CAD build for the part. Positions are in the model's coordinates, mm. Round coordinates to 2 decimals unless told otherwise and drop trailing zeros. Loops run counter-clockwise (first coordinate to the right, second up) from the corner with the lowest first, then second, coordinate; pieces in that order, holes last. Notation, with made-up numbers: M 50,-13 L 94,-13 A24 cw 94,4 Z; hole C -14,-8.5 d2. An arc over 180 degrees is marked long. Put each result on its own line as item: value. Start each with the question number.
from build123d import *

# Parameters (mm, degrees)
SKETCH1_W           = 8.5
SKETCH1_H           = 8
BOSS_EXTRUDE1_DEPTH = 4.2
CUT_EXTRUDE1_DEPTH  = 14.2
CHAMFER1_SIZE       = 1.090756547
CHAMFER1_SIZE_2     = 1
FILLET1_R           = 1
FILLET2_R           = 0.2
FILLET3_R           = 0.02
SKETCH3_R           = 0.5
CUT_EXTRUDE2_DEPTH  = 14.2
CHAMFER2_SIZE       = 0.1


with BuildPart() as part:
    # Sketch1 → Boss-Extrude1 (new body)
    with BuildSketch(Plane(origin=(0, 0, 0), x_dir=(1, 0, 0), z_dir=(0, 1, 0))):
        Rectangle(SKETCH1_W, SKETCH1_H)
    extrude(amount=BOSS_EXTRUDE1_DEPTH)

    # Sketch2 → Cut-Extrude1 (cut)
    with BuildSketch(Plane(origin=(4.25, 0, 0), x_dir=(0, 0, -1), z_dir=(1, 0, 0))):
        with BuildLine():
            Line((-4, 3.9), (-5.253535024, 5.241651662))
            Line((-5.253535024, 5.241651662), (3.889156526, 7.141243929))
            Line((3.889156526, 7.141243929), (5.679183493, 5.077233243))
            Line((5.679183493, 5.077233243), (4, 3.9))
            ThreePointArc((4, 3.9), (0, 4.060256822), (-4, 3.9))
        make_face()
        with BuildLine():
            Line((4.717394395, 0), (0, -2.904825783))
            Line((0, -2.904825783), (-4.70037365, 0))
            ThreePointArc((-4.70037365, 0), (0.008510373, 0.222229748), (4.717394395, 0))
        make_face()
    extrude(amount=-CUT_EXTRUDE1_DEPTH, mode=Mode.SUBTRACT)

    # Chamfer1
    # the kernel refuses this chamfer: 1.090756547, 1 mm, written as the material it takes off along each edge
    with BuildSketch(Plane(origin=(7.060832105, 3.9, -4), x_dir=(0, -1, 0), z_dir=(-1, 0, 0))) as chamfer1_piece_1:
        with BuildLine():
            Line((CHAMFER1_SIZE, 0), (-0.069441157, 0.98780495))
            ThreePointArc((-0.069441157, 0.98780495), (-0.038234412, 0.508961249), (0, 0))
            Line((0, 0), (CHAMFER1_SIZE, 0))
        make_face()
    extrude(amount=14.12166421, mode=Mode.SUBTRACT)
    with BuildSketch(Plane(origin=(7.026184696, 3.9, 4), x_dir=(0, 0.06925797782051132, -0.9975987833333668), z_dir=(-1, 0, 0))) as chamfer1_piece_2:
        with BuildLine():
            Line((1.077190612, 0), (-CHAMFER1_SIZE_2 * 0.0692579778205, CHAMFER1_SIZE_2 * 0.997598783333))
            Line((-CHAMFER1_SIZE_2 * 0.0692579778205, CHAMFER1_SIZE_2 * 0.997598783333), (0, 0))
            ThreePointArc((0, 0), (0.555048482, -0.002898226), (1.077190612, 0))
        make_face()
    extrude(amount=14.052369392, mode=Mode.SUBTRACT)

    # Fillet1
    fillet1_edges = [part.edges().sort_by_distance(p)[0] for p in [
        (0, 0.062655213, -4),
        (0, 0.061289175, 4),
    ]]
    fillet(fillet1_edges, radius=FILLET1_R)

    # Fillet2
    fillet2_edges = [part.edges().sort_by_distance(p)[0] for p in [
        (0, 2.809243453, -4),
        (0, 3.974604043, 2.925395957),
        (0, 3.969441157, -3.01219505),
        (0, 2.9, 4),
    ]]
    fillet(fillet2_edges, radius=FILLET2_R)

    # Fillet3
    fillet3_edges = [part.edges().sort_by_distance(p)[0] for p in [
        (4.25, 0.222229049, -0.000152397),
        (4.25, 0.406869221, -3.686055151),
        (4.25, 0.405751593, 3.685933525),
        (-4.25, 0.222229049, -0.000152397),
        (-4.25, 0.406869221, -3.686055151),
        (-4.25, 0.405751593, 3.685933525),
        (4.25, 1.93502694, -4),
        (-4.25, 1.93502694, -4),
        (4.25, 1.975286544, 4),
        (4.25, 3.384901314, -3.509878633),
        (4.25, 4.060241686, -0.03890618),
        (4.25, 3.439667659, 3.460332341),
        (4.25, 2.893693974, 3.984775907),
        (4.25, 3.961854563, 2.919594368),
        (4.25, 3.953888859, -3.004346497),
        (4.25, 2.804713491, -3.987691713),
        (-4.25, 3.384901314, -3.509878633),
        (-4.25, 1.975286544, 4),
        (-4.25, 3.439667659, 3.460332341),
        (-4.25, 4.060241686, -0.03890618),
        (-4.25, 2.893693974, 3.984775907),
        (-4.25, 3.961854563, 2.919594368),
        (-4.25, 3.953888859, -3.004346497),
        (-4.25, 2.804713491, -3.987691713),
    ]]
    fillet(fillet3_edges, radius=FILLET3_R)

    # Sketch3 → Cut-Extrude2 (cut)
    with BuildSketch(Plane.ZY.offset(4.25)):
        with Locations((-1.55, 1.4)):
            Circle(SKETCH3_R)
        with Locations((1.55, 1.4)):
            Circle(SKETCH3_R)
    extrude(amount=-CUT_EXTRUDE2_DEPTH, mode=Mode.SUBTRACT)

    # Chamfer2
    chamfer2_edges = [part.edges().sort_by_distance(p)[0] for p in [
        (4.25, 1.4, -2.05),
        (-4.25, 1.4, -2.05),
        (4.25, 1.4, 1.05),
        (-4.25, 1.4, 1.05),
    ]]
    chamfer(chamfer2_edges, length=CHAMFER2_SIZE)


solid = part.part
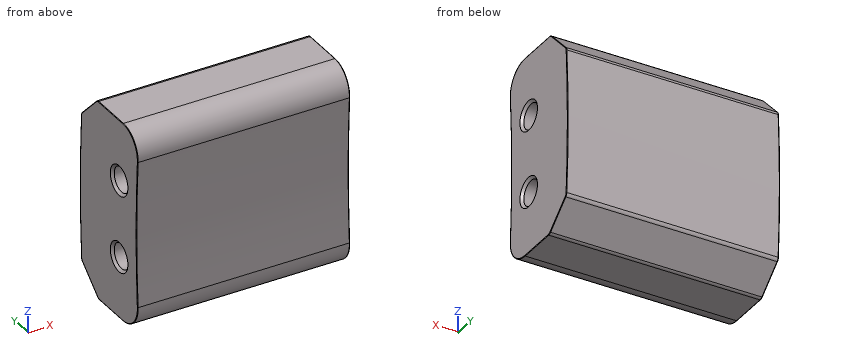
(1) Cut at A-A on y = 1.4. Count the separate pieces of the cut face and the enclosed holes in it, and give its area (3 significant figures).
(2) Cut at B-B on x = -3.25. List the corners of the cut face in (y, z), and give its area (3 significant figures).
(3) Drill centre lines: line 1 along Z through (x, y) = (2.25, 1.3); line 2 along Y through (x, z) = (1, -0.25); line 3 along Y through (x, z) = (0.75, -1.55). Where is each one in solid material? Low to high.
Taken from the geometry:
1. separate pieces: 3
1. enclosed holes: 0
1. area: 51.0 mm2
2. outline: M 0.14,-2.94 A1 ccw 1.13,-4 L 2.74,-4 A0.2 ccw 2.87,-3.95 L 3.9,-3.07 A0.2 ccw 3.97,-2.93 A50 ccw 3.98,2.85 A0.2 ccw 3.92,2.98 L 2.96,3.94 A0.2 ccw 2.82,4 L 1.13,4 A1 ccw 0.14,2.94 A50 cw Z; hole C 1.4,-1.55 d1; hole C 1.4,1.55 d1
2. area: 27.6 mm2
3. line 1: -4 to -2.04, -1.06 to 1.06, 2.04 to 4
3. line 2: 0.22 to 4.06
3. line 3: 0.2 to 0.9, 1.9 to 4.04
